Input: part model. Units: mm. Frame: model coordinates. A direction names the side the tool comes from. Round coordinates to 2 decimals unless told otherwise and drop trailing zeros. Loops run counter-clockwise (first coordinate to the right, second up) from the corner with the lowest first, then second, coordinate; pieces in that order, holes last.
1) First-contact query: pin 1 (1.5 mm diameter, centred on y = -0.5, z = 6, fed in from +X); pin 2 (1 mm diameter, centred on y = 6, z = 2.5, fed in from +X); pin 3 (4 mm diameter, centred on x = 0, y = 0, fed in from -Z); pin 4 (1.5 mm diameter, centred on x = -1.5, y = 3.5, fed in from -Z). Flat tips, straight axial feed; report the tip coordinate or a pass-through.
2) Section B-B, the plane y = 0. Return loops of the section in (x, z), and give its area (3 significant figures).
3) Ray query, line 1 along X through (y, z) = (-1.75, 4.25); line 2 along Y through (x, z) = (0.25, 3); line 3 along Z through (x, y) = (-1.5, -5.5). Return the intervals inside material, ascending.
4) Access query for faces 4 (the face through (-2.43, 4.288, 6.479)), 5 (the face through (0, 0, 5)), 6 (the face through (2.43, -4.288, 6.479)). Directions: +Z, -Z, +X, -X, +Y, -Y. A direction counts if a zero-diameter tool reaches every point of the face in a straight line with its end or side. Return the directions, or none.
5) Section D-D, the plane z = 7.25. Return loops of the section in (x, y).
6) Section C-C, the plane x = 3.75. Return loops of the section in (y, z), and give its area (3 significant figures).
7) Draft query along X for faces 1 (the face through (-2.499, -4.248, 6.479)), 2 (the face through (2.499, 4.248, 6.479)), 3 (the face through (0.54, -2.44, 2.97)). Return one class per face: pulls with the +X half, pulls with the -X half, needs draft (parallel to the pull), parting line crosses it, or undercut.
8) Section A-A, the plane z = 1.75. Return loops of the section in (x, y), and give its area (3 significant figures).
Autodesk Inventor part; units mm, degrees
ref_plane "YZ Plane" through (0, 0, 0) normal (1, 0, 0) x (0, 1, 0)
ref_plane "XZ Plane" through (0, 0, 0) normal (0, 1, 0) x (-1, 0, 0)
ref_plane "XY Plane" through (0, 0, 0) normal (0, 0, 1) x (1, 0, 0)
sketch "Sketch1" plane through (0, 0, 0) normal (0, 0, 1) x (1, 0, 0)
  line L0 (0, 8) -> (6.9282, 4)
  line L1 (6.9282, 4) -> (6.9282, -4)
  line L2 (6.9282, -4) -> (0, -8)
  line L3 (0, -8) -> (-6.9282, -4)
  line L4 (-6.9282, -4) -> (-6.9282, 4)
  line L5 (-6.9282, 4) -> (0, 8)
  point P0 (0, 0)
  point P1 (0, 0)
  dimension "d0" = 8
extrude "Extrusion1" add sketch "Sketch1" along normal blind 5
sketch "Sketch2" plane through (0, 0, 5) normal (0, 0, 1) x (1, 0, 0)
  line L0 (-6.9282, 4) -> (-6.9282, -4)
  line L1 (-6.9282, -4) -> (0, -8)
  line L2 (0, -8) -> (6.9282, -4)
  line L3 (6.9282, -4) -> (6.9282, 4)
  line L4 (6.9282, 4) -> (0, 8)
  line L5 (0, 8) -> (-6.9282, 4)
  line L6 (-4.9282, 2.8453) -> (-4.9282, -2.8453)
  line L7 (-4.9282, -2.8453) -> (0, -5.6906)
  line L8 (0, -5.6906) -> (4.9282, -2.8453)
  line L9 (4.9282, -2.8453) -> (4.9282, 2.8453)
  line L10 (4.9282, 2.8453) -> (0, 5.6906)
  line L11 (0, 5.6906) -> (-4.9282, 2.8453)
  point P0 (0, 0)
  dimension "d3" = 2
extrude "Extrusion2" add sketch "Sketch2" along normal blind 3 contours L11 L10 L9 L8 L7 L6
sketch "Sketch3" plane through (0, 0, 0) normal (0, 0, -1) x (-1, 0, 0)
  circle A0 centre (0, 0) radius 2.5
  dimension "d6" = 5
extrude "Extrusion3" cut sketch "Sketch3" against normal blind 5
chamfer "Chamfer1" distance 1 angle 45 1 edges at (2.5, 0, 0)
properties part number "white_part1"
Final values:
1. pin 1: stops at x = 4.93
1. pin 2: stops at x = 4.33
1. pin 3: stops at z = 5
1. pin 4: stops at z = 0
2. outline: (-6.93, 0) - (-3.5, 0) - (-2.5, 1) - (-2.5, 5) - (2.5, 5) - (2.5, 1) - (3.5, 0) - (6.93, 0) - (6.93, 5) - (4.93, 5) - (4.93, 8) - (-4.93, 8) - (-4.93, 5) - (-6.93, 5) - close
2. area: 72.9 mm2
3. line 1: x = -6.93 to -1.79, 1.79 to 6.93
3. line 2: y = -7.86 to -2.49, 2.49 to 7.86
3. line 3: z = 0 to 5
4. face 4: +Z, -X, +Y
4. face 5: -Z
4. face 6: +Z, +X, -Y
5. outline: (-4.93, -2.85) - (0, -5.69) - (4.93, -2.85) - (4.93, 2.85) - (0, 5.69) - (-4.93, 2.85) - close
6. outline: (-5.83, 0) - (5.83, 0) - (5.83, 5) - (3.53, 5) - (3.53, 8) - (-3.53, 8) - (-3.53, 5) - (-5.83, 5) - close
6. area: 79.5 mm2
7. face 1: pulls with the -X half
7. face 2: pulls with the +X half
7. face 3: undercut
8. outline: (-6.93, -4) - (0, -8) - (6.93, -4) - (6.93, 4) - (0, 8) - (-6.93, 4) - close; hole circle Ø5 at (0, 0)
8. area: 147 mm2
